Input: part model. Units: mm. Frame: model coordinates. Face numbers are marked on the shaded views. Give positions to 0.01 mm unless a question says otherwise; leave off trailing zeros. Loops run counter-clockwise (first coordinate to the right, second up) from the corner with the lowest first, then second, coordinate; pieces in that order, holes last. Notation, with made-up numbers: M 71,76.25 L 96,76.25 A24 ccw 96,107.25 Z; hole C 48,-6 d4. An arc over 180 degrees is marked long. Return JSON: item names as keys, results as strings. Group by question number.
Autodesk Inventor part; units mm, degrees
ref_plane "YZ Plane" through (0, 0, 0) normal (1, 0, 0) x (0, 1, 0)
ref_plane "XZ Plane" through (0, 0, 0) normal (0, 1, 0) x (-1, 0, 0)
ref_plane "XY Plane" through (0, 0, 0) normal (0, 0, 1) x (1, 0, 0)
ref_plane "Work Plane12" through (10, 45.7, 9.8) normal (0, -1, 0) x (1, 0, 0)
sketch "Sketch20" plane through (10, 45.7, 9.8) normal (0, -1, 0) x (1, 0, 0)
  circle A0 centre (0, 10.22) radius 1.15
  circle A1 centre (0, 13.22) radius 1.15
  circle A2 centre (0, 7.22) radius 1.15
  circle A3 centre (0, 16.22) radius 1.15
  arc A4 (2.55, 20.12) -> (-2.55, 20.12) centre (0, 19.8141) ccw
  line L0 (-2.55, 20.12) -> (-4.4453, 4.3219)
  arc A5 (-4.4453, 4.3219) -> (4.4453, 4.3219) centre (0, 0) ccw
  line L1 (4.4453, 4.3219) -> (2.55, 20.12)
  circle A6 centre (0, 0) radius 1.65
  arc A7 (2.1528, 20.0724) -> (-2.1528, 20.0724) centre (0, 19.8141) ccw
  line L2 (-2.1528, 20.0724) -> (-4.0646, 4.1375)
  arc A8 (-4.0646, 4.1375) -> (4.0646, 4.1375) centre (0, 0) ccw
  line L3 (4.0646, 4.1375) -> (2.1528, 20.0724)
  point P0 (-10, -9.8)
  dimension "d95" = 0.4
extrude "Extrusion21" add sketch "Sketch20" along normal blind 3 contours L3 A8 L2 A7
properties part number "X4_leg_Servo_horn" material "Default New Material"
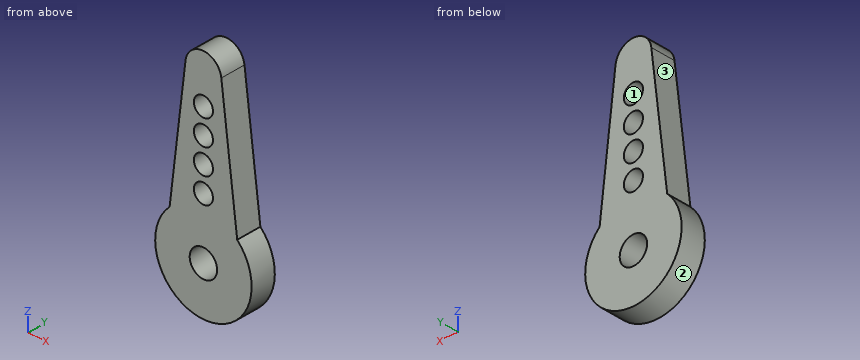
Item 1: Section A-A, the plane z = 9.8. Return loops of the section in (x, y), then the cut area to 3 significant figures.
Item 2: Section B-B, the plane y = 45.25. Return loops of the section in (x, z), then the cut area to 3 significant figures.
Item 3: Section D-D, the plane z = 19.5. Return loops of the section in (x, y), then the cut area to 3 significant figures.
Item 4: Material intervals for line 1 (Z direction, x = 10.75, y = 45.4); line 2 (Z direction, x = 11.25, y = 42.9); line 3 (X direction, y = 43.8, z = 17), sorted ascending. Write a range as from..to.
Item 5: Section C-C, the plane x = 10. Return loops of the section in (y, z).
Item 6: Pull-direction query (X, two-part tool) for the marked faces 1, 2 and 3; classes: pulls with the +X half, pulls with the -X half, needs draft (parallel to the pull), parting line crosses it, or undercut.
Answer below:
{
 "1": {"outline": "M 4.2,42.7 L 8.35,42.7 L 8.35,45.7 L 4.2,45.7 Z; M 11.65,42.7 L 15.8,42.7 L 15.8,45.7 L 11.65,45.7 Z", "area": "24.9 mm^2"},
 "2": {"outline": "M 5.94,13.94 A5.8 ccw long 14.06,13.94 L 12.15,29.87 A2.17 ccw 7.85,29.87 Z; hole C 10,9.8 d3.3; hole C 10,17.02 d2.3; hole C 10,20.02 d2.3; hole C 10,23.02 d2.3; hole C 10,26.02 d2.3", "area": "177 mm^2"},
 "3": {"outline": "M 6.6,42.7 L 8.97,42.7 L 8.97,45.7 L 6.6,45.7 Z; M 11.03,42.7 L 13.4,42.7 L 13.4,45.7 L 11.03,45.7 Z", "area": "14.2 mm^2"},
 "4": {"line 1": "4.05..8.33, 11.27..16.15, 17.89..19.15, 20.89..22.15, 23.89..25.15, 26.89..31.65", "line 2": "4.14..8.72, 10.88..31.39", "line 3": "6.3..8.85, 11.15..13.7"},
 "5": {"outline": "M 42.7,4 L 45.7,4 L 45.7,8.15 L 42.7,8.15 Z; M 42.7,11.45 L 45.7,11.45 L 45.7,15.87 L 42.7,15.87 Z; M 42.7,18.17 L 45.7,18.17 L 45.7,18.87 L 42.7,18.87 Z; M 42.7,21.17 L 45.7,21.17 L 45.7,21.87 L 42.7,21.87 Z; M 42.7,24.17 L 45.7,24.17 L 45.7,24.87 L 42.7,24.87 Z; M 42.7,27.17 L 45.7,27.17 L 45.7,31.78 L 42.7,31.78 Z"},
 "6": {"face 1": "undercut", "face 2": "parting line crosses it", "face 3": "pulls with the -X half"}
}
